Verification items for the finished model (mm, model axes). A direction names the side the tool comes from. Round coordinates to 2 decimals unless told otherwise and drop trailing zeros. Write each loop counter-clockwise with the first axis right and the second up, starting at its lowest first coordinate (ties: lowest second). Pieces come first, ordered by that corner, then holes. Notation, with made-up numbers: M 76.5,-18.5 L 130.5,-18.5 A30 ccw 130.5,3.5 Z; hole C 59,-31.5 d3. An arc over 180 degrees is marked long. Write each question's results on one line, items separated by ' | '.
from build123d import *

# Parameters (mm, degrees)
F0_R     = 4.25
F0_W     = 8
F0_H     = 15
F1_DEPTH = 5


# Not quite as in the source:
# - a feature names something its author has since deleted; it is built from what else it names


with BuildPart() as f1:
    # F0 (on Right) → F1 (new body)
    with BuildSketch(Plane.YZ):
        with BuildLine():
            Line((-7.5, -10), (7.5, -10))
            ThreePointArc((7.5, -10), (11.5869510213, 4.689623229), (-1.5666059757, 12.4014412758))
            ThreePointArc((-1.5666059757, 12.4014412758), (-12.0833347544, 3.2004720296), (-7.5, -10))
        make_face()
        Circle(F0_R, mode=Mode.SUBTRACT)
        with BuildLine():
            ThreePointArc((-1.5666059757, 12.4014412758), (11.5869510213, 4.689623229), (7.5, -10))
            Line((7.5, -10), (13.9559781345, -10))
            Line((13.9559781345, -10), (40, -5))
            Line((40, -5), (40, 0))
            Line((40, 0), (40, 15))
            Line((40, 15), (40, 20))
            Line((40, 20), (-1.5666059757, 12.4014412758))
        make_face()
        with Locations((44, 7.5)):
            Rectangle(F0_W, F0_H)
    extrude(amount=F1_DEPTH)


solid = f1.part
1) Sectioned sample at D-D, the plane y = 35. Record the cut outline in (x, z), and give its area (3 significant figures).
Calculated:
outline: M 0,-5.96 L 5,-5.96 L 5,19.09 L 0,19.09 Z | area: 125 mm²
2) Access from +Z, -Z, +X, -X, +Y, -Y to the whole of each face (thin tool, end or side, straight path). Record for faces 4 (the flat face through (2, 40, -3)), 5 (the flat face through (2, 48, 7)), 6 (the flat face through (2, 40, 17)).
Calculated:
face 4: -Z, +X, -X, +Y | face 5: +Z, -Z, +X, -X, +Y | face 6: +Z, +X, -X, +Y
3) Material ranges on line 1 (Z direction, x = 1.3, y = 42.5); line 2 (Y direction, x = 1.25, z = 3.75); line 3 (Z direction, x = 2.95, y = 0), recorded low to high. Write a range as [from, to].
Calculated:
line 1: z = [0, 15] | line 2: y = [-11.92, -2], [2, 48] | line 3: z = [-10, -4.25], [4.25, 12.69]
4) Sectioned sample at B-B, the plane x = 2.85. Record the cut outline in (y, z).
Calculated:
outline: M -7.5,-10 L 13.96,-10 L 40,-5 L 40,0 L 48,0 L 48,15 L 40,15 L 40,20 L -1.57,12.4 A12.5 ccw Z; hole C 0,0 d8.5
5) Draft check along Z on faces 1 (the flat face through (2, 44, 0)), 2 (the flat face through (5, 17, 5)), 3 (the cylindrical face through (2.465, 2.285, 3.584)). Enter one of: pulls with the +Z half, pulls with the -Z half, needs draft (parallel to the pull), parting line crosses it, or undercut.
Calculated:
face 1: pulls with the -Z half | face 2: needs draft | face 3: undercut
6) Sectioned sample at C-C, the plane y = 0. Record the cut outline in (x, z).
Calculated:
outline: M 0,-10 L 5,-10 L 5,-4.25 L 0,-4.25 Z; M 0,4.25 L 5,4.25 L 5,12.69 L 0,12.69 Z
7) Sectioned sample at A-A, the plane z = 3.5. Record the cut outline in (x, y).
Calculated:
outline: M 0,-12 L 5,-12 L 5,-2.41 L 0,-2.41 Z; M 0,2.41 L 5,2.41 L 5,48 L 0,48 Z
8) Depth check by flat-ended pin: P1, Ø1.5, axis at x = 2, z = 16.5, coming from the +Y side; P2, Ø2.5, axis at x = 1.5, y = 45, coming from the -Z side; P3, Ø7, axis at y = 0, z = 0, coming from the +X side. Enter the tip coordinate at first touch or a pass-through.
Calculated:
P1: stops at y = 40 | P2: stops at z = 0 | P3: passes through
